Read the model definition and answer for the solid it produces. Units are mm, in the model's axes. A direction names the side the tool comes from. Give positions to 0.01 mm unless a question says otherwise; leave off trailing zeros. Order: outer loops, then holes, each group sorted by start corner. A loop starts at its lowest first (then second) coordinate and runs counter-clockwise, first axis right, second up. Notation, with made-up numbers: M 49,62 L 53,62 A19 ccw 53,89 Z; hole C -27,80.5 d5. An arc over 180 degrees is marked long. Write item = value, one per line. Start each with the question number.
Autodesk Inventor part; units mm, degrees
ref_plane "YZ Plane" through (0, 0, 0) normal (1, 0, 0) x (0, 1, 0)
ref_plane "XZ Plane" through (0, 0, 0) normal (0, 1, 0) x (-1, 0, 0)
ref_plane "XY Plane" through (0, 0, 0) normal (0, 0, 1) x (1, 0, 0)
sketch "Boceto1" plane through (0, 0, 0) normal (1, 0, 0) x (0, 1, 0)
  line L0 (0, 0) -> (0, 60)
  line L1 (0, 0) -> (0, -80)
  line L2 (0, 60) -> (3, 60)
  line L3 (3, -80) -> (0, -80)
  line L4 (3, 60) -> (53, 60)
  line L5 (53, 60) -> (53, 57)
  line L6 (53, 57) -> (3, 57)
  line L7 (3, 32) -> (53, 32)
  line L8 (53, 32) -> (53, 29)
  line L9 (53, 29) -> (3, 29)
  line L10 (3, 57) -> (3, 32)
  line L11 (3, 29) -> (3, -80)
  dimension "d0" = 60
  dimension "d1" = 80
  dimension "d2" = 3
  dimension "d3" = 140
  dimension "d4" = 50
  dimension "d5" = 3
  dimension "d6" = 50
  dimension "d7" = 3
  dimension "d8" = 25
extrude "Extrusión1" add sketch "Boceto1" against normal blind 40
sketch "Boceto2" plane through (0, 3, 29) normal (0, 1, 0) x (1, 0, 0)
  line L0 (-40, 109) -> (-40, -31)
  line L1 (0, 109) -> (-40, 109)
  arc A0 (0, 89) -> (-40, 89) centre (-20, 89) ccw
  line L2 (0, 89) -> (0, 109)
  line L3 (-40, 109) -> (-40, 89)
  point P0 (0, 29)
  point P1 (-20, 109)
extrude "Extrusión2" cut sketch "Boceto2" against normal blind 40
sketch "Boceto3" plane through (0, 0, 60) normal (0, 0, 1) x (1, 0, 0)
  line L0 (0, 53) -> (-40, 53)
  arc A0 (0, 33) -> (-40, 33) centre (-20, 33) ccw
  line L1 (-40, 33) -> (-40, 53)
  line L2 (0, 53) -> (0, 33)
  point P0 (0, 0)
  point P1 (-20, 53)
extrude "Extrusión3" cut sketch "Boceto3" against normal blind 40
sketch "Boceto4" plane through (-40, 0, 60) normal (0, 0, 1) x (1, 0, 0)
  arc A0 (40, 33) -> (0, 33) centre (20, 33) ccw
  circle A1 centre (20, 33) radius 4
  point P0 (40, 0)
  dimension "d15" = 8
extrude "Extrusión4" cut sketch "Boceto4" against normal blind 40
sketch "Boceto5" plane through (-40, 3, 29) normal (0, 1, 0) x (1, 0, 0)
  line L0 (0, 0) -> (0, 89.224)
  line L1 (0, 44.612) -> (40, 44.612)
  line L2 (20, 44.612) -> (20, 54.612)
  circle A0 centre (20, 54.612) radius 5
  point P0 (40, 29)
  dimension "d20" = 10
  dimension "d21" = 10
extrude "Extrusión5" cut sketch "Boceto5" against normal blind 40
sketch "Boceto6" plane through (-40, 3, 29) normal (0, 1, 0) x (1, 0, 0)
  line L0 (27.5, 62.112) -> (12.5, 62.112)
  line L1 (12.5, 62.112) -> (12.5, 47.112)
  line L2 (12.5, 47.112) -> (27.5, 47.112)
  line L3 (27.5, 47.112) -> (27.5, 62.112)
  circle A0 centre (20, 54.612) radius 5
  line L4 (27.5, 62.112) -> (12.5, 47.112) construction
  line L5 (12.5, 62.112) -> (27.5, 47.112) construction
  circle A1 centre (12.5, 62.112) radius 1.5
  circle A2 centre (27.5, 62.112) radius 1.5
  circle A3 centre (12.5, 47.112) radius 1.5
  circle A4 centre (27.5, 47.112) radius 1.5
  point P0 (40, 29)
  dimension "d24" = 15
  dimension "d25" = 15
  dimension "d26" = 3
  dimension "d27" = 3
  dimension "d28" = 3
  dimension "d29" = 3
extrude "Extrusión6" cut sketch "Boceto6" against normal blind 5 contours A1 L1 L0 | L0 L1 A1 | A2 L3 L0 | L0 L3 A2 | A3 L2 L1 | L1 L2 A3 | A4 L2 L3 | L3 L2 A4
properties part number "Base_engine" material "Plástico ABS"
1) Find the intervals of material crossed by probe 1 along Z at (x, y) = (-19.5, 38.5); probe 2 along Y at (x, z) = (-20, 31.1); probe 3 along Z at (x, y) = (-27, 2) (3 decimals), in increasing order. Write a range as [from, to].
2) For a pull along X with two mould halves and no side action, classify faces 4 (the face through (-23.685, 1.521, -28.991)), 5 (the face through (-20, 53, 31)), 6 (the face through (-20, 28, 57)) as pulls with the +X half, pulls with the -X half, needs draft (parallel to the pull), parting line crosses it, or undercut.
3) For faces 1 (the face through (-11, 3, -25)), 2 (the face through (-20, 28, 32)), 3 (the face through (-27.83, 1.52, -31.65)), determine the directions among +Z, -Z, +X, -X, +Y, -Y from which every point of the face is accessible in a straight line to the end or side of a thin tool.
4) Find section B-B on y = 16. Determine the outline of the cut face in (x, z), plus the area to 3 significant figures.
5) Find section D-D on y = 42. Determine the outline of the cut face in (x, z), plus the area to 3 significant figures.
6) Find section C-C on x = -27.5. Determine the outline of the cut face in (y, z).
7) Each of these flat-tipped pins is pushed along its axis until it touches: P1, Ø12, axis at x = -24, y = 36.5, coming from the -Z side; P2, Ø13, axis at x = -20, y = 33, coming from the +Z side; P3, Ø12, axis at x = -20, z = -29.5, coming from the +Y side. Where does it stop, or does it pass through?
8) Find section A-A on x = -20. Determine the outline of the cut face in (y, z), plus the area to 3 significant figures.
Numbers:
q1.probe_1 = [29, 32], [57, 60]
q1.probe_2 = [0, 29], [37, 53]
q1.probe_3 = [-78.735, -34.526], [-31.698, -19.526], [-16.698, 60]
q2.face_4 = undercut
q2.face_5 = parting line crosses it
q2.face_6 = needs draft
q3.face_1 = -Z, +X, -X, +Y
q3.face_2 = +X, -X, +Y
q3.face_3 = +Y, -Y
q4.outline = M -40,29 L 0,29 L 0,32 L -40,32 Z; M -40,57 L 0,57 L 0,60 L -40,60 Z
q4.area = 240 mm2
q5.outline = M -37.86,29 L -2.14,29 L -2.14,32 L -37.86,32 Z; M -37.86,57 L -2.14,57 L -2.14,60 L -37.86,60 Z
q5.area = 214 mm2
q6.outline = M 0,-78.54 L 3,-78.54 L 3,-34.61 L 0,-34.61 Z; M 0,-31.61 L 3,-31.61 L 3,-19.61 L 0,-19.61 Z; M 0,-16.61 L 3,-16.61 L 3,29 L 51.54,29 L 51.54,32 L 3,32 L 3,57 L 51.54,57 L 51.54,60 L 0,60 Z
q7.P1 = 29
q7.P2 = 60
q7.P3 = 3
q8.outline = M 0,-80 L 3,-80 L 3,-30.61 L 0,-30.61 Z; M 0,-20.61 L 3,-20.61 L 3,29 L 29,29 L 29,32 L 3,32 L 3,57 L 29,57 L 29,60 L 0,60 Z; M 37,29 L 53,29 L 53,32 L 37,32 Z; M 37,57 L 53,57 L 53,60 L 37,60 Z
q8.area = 642 mm2
